```python
from build123d import *


with BuildPart() as part:
    # Sketch3 → Revolve1 (revolve)
    with BuildSketch(Plane.XY):
        with BuildLine():
            Line((-41.971552217, 86.483404529), (-54.944062896, 0))
            Line((-54.944062896, 0), (-60, 0))
            Line((-60, 0), (-30, 200))
            Line((-30, 200), (0, 200))
            Line((0, 200), (0, 195))
            Line((0, 195), (-17.082188688, 195))
            ThreePointArc((-17.082188688, 195), (-23.607752062, 192.577402104), (-26.971552217, 186.483404529))
            Line((-26.971552217, 186.483404529), (-41.971552217, 86.483404529))
        make_face()
    revolve(axis=Axis((0, 0, 0), (0, 1, 0)))


solid = part.part
```
Design review of the part built by this model. Coordinates are the model's own, in mm. Give positions to 0.01 mm unless a question says otherwise; leave off trailing zeros. Order: outer loops, then holes, each group sorted by start corner. A loop starts at its lowest first (then second) coordinate and runs counter-clockwise, first axis right, second up. Notation, with made-up numbers: M -27.5,66.5 L 9.5,66.5 A16 ccw 9.5,91.5 Z; hole C 18.25,-22.5 d6. An arc over 180 degrees is marked long. One line per question, with ' | ' between items. Start each with the question number.
Q1. We need section B-B (y = 183.5). Write out the cut boundary in (x, z) (3 decimals), plus the area to 3 significant figures.
Q2. The part is to be moulded in two halves that separate along X. For faces 1 (the face through (26, 0, -49)), 2 (the face through (0, 195, 0)), 3 (the face through (-42.722, 101.4, 13.454)), say which applies: +X half, -X half, draft (parallel to the pull), parting line (faces both ways), or undercut.
Q3. For L1, parallel to X at y = 20, z = -47; L2, parallel to X at y = 59.5, z = -32; L3, parallel to Z at x = 2, y = 23.5, list the stretches that pass through material, from the lowest coordinate up. Write a range as [from, to].
Q4. We need section A-A (y = 147). Write out the cut boundary in (x, z), plus the area to 3 significant figures.
Q5. For pin 1 Ø17 at (x, z) = (4, -4.5) entering from -Y; pin 2 Ø1 at (y, z) = (151, 26.5) entering from -X; pin 3 Ø1.5 at (y, z) = (127.5, 29.5) entering from -X, all flat-tipped, find the tip position at first contact; note any pin that passes through.
Returned:
1) outline: C 0,0 d64.95; hole C 0,0 d54.838 | area: 951 mm2
2) face 1: draft | face 2: undercut | face 3: parting line
3) L1: [-32.25, -22.12], [22.12, 32.25] | L2: [-39.81, -33.07], [33.07, 39.81] | L3: [-56.44, -51.38], [51.38, 56.44]
4) outline: C 0,0 d75.9; hole C 0,0 d65.79 | area: 1,130 mm2
5) pin 1: y = 195 | pin 2: x = -26.83 | pin 3: x = -29.07
